Design review of the part shown in the three views and the two pictorial views. Dimensions are in mm from the part's minimum x, y and z. Give positions to 0.01 mm unless a question says otherwise; leave off trailing zeros. Order: outer loops, then holes, each group sorted by start corner. A loop starts at its lowest first (then second) coordinate and runs counter-clockwise, first axis right, second up. Notation, with made-up numbers: (83.25, 79) -> (142.25, 79) arc R4 ccw to (142.25, 84) -> close; hole circle Ø11 at (-23.75, 81). An arc over 180 degrees is marked (long way). Use one line per item in the form item = value.
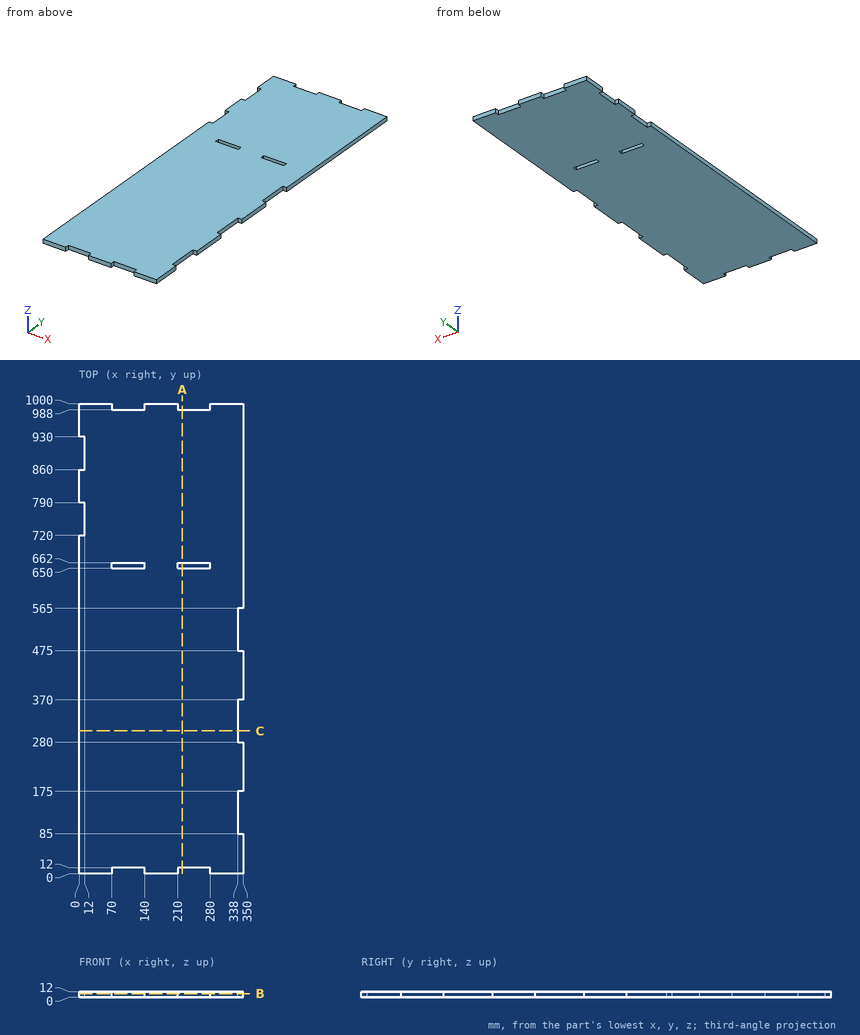
1. Add section B-B on z = 8. Count the separate pieces of the cut face and the enclosed holes in it, then the cut area to 3 significant figures.
Values:
separate_pieces = 1
enclosed_holes = 2
area = 340,000 mm^2
2. For L1, parallel to Y at x = 122.5, z = 2; L2, parallel to X at y = 789, z = 2; L3, parallel to X at y = 319, z = 4.25, list the stretches that pass through material, from the lowest coordinate up.
Values:
L1 = 12 to 650, 662 to 988
L2 = 12 to 350
L3 = 0 to 338
3. Add section A-A on x = 220. Give the boundary of the cut face in (y, z), then the cut area to 3 significant figures.
Values:
outline = (12, 0) -> (650, 0) -> (650, 12) -> (12, 12) -> close; (662, 0) -> (988, 0) -> (988, 12) -> (662, 12) -> close
area = 11,600 mm^2
4. Add section C-C on y = 304. Give the boundary of the cut face in (x, z), then the cut area to 3 significant figures.
Values:
outline = (0, 0) -> (338, 0) -> (338, 12) -> (0, 12) -> close
area = 4,060 mm^2
5. For pin 1 Ø1 at (x, z) = (102.5, 7) entering from -Y, flat-tipped, find the tip position at first contact; note if it passes through.
Values:
pin_1 = 12
